```python
from build123d import *

# Parameters (mm, degrees)
BOSS_EXTRUDE1_DEPTH = 2
CHAMFER3_SIZE       = 0.2
SKETCH4_R           = 1
SKETCH4_R_2         = 2
CUT_EXTRUDE3_DEPTH  = 2
CHAMFER5_SIZE       = 0.1
CHAMFER6_SIZE       = 0.1


with BuildPart() as part:
    # Sketch1 → Boss-Extrude1 (new body)
    with BuildSketch(Plane.XY):
        with BuildLine():
            Line((-18, 3), (18, 3))
            ThreePointArc((18, 3), (21, 0), (18, -3))
            Line((18, -3), (-18, -3))
            ThreePointArc((-18, -3), (-21, 0), (-18, 3))
        make_face()
    extrude(amount=BOSS_EXTRUDE1_DEPTH)

    # Chamfer3
    chamfer3_edges = [part.edges().sort_by_distance(p)[0] for p in [
        (21, 0, 2),
        (0, 3, 2),
        (-21, 0, 2),
        (0, 3, 0),
        (21, 0, 0),
        (0, -3, 0),
        (-21, 0, 0),
        (0, -3, 2),
    ]]
    chamfer(chamfer3_edges, length=CHAMFER3_SIZE)

    # Sketch4 → Cut-Extrude3 (cut)
    with BuildSketch(Plane.XY.offset(2)):
        with Locations((-18, 0)):
            Circle(SKETCH4_R)
        with Locations((-12, 0)):
            Circle(SKETCH4_R_2)
        with Locations((-4, 0)):
            Circle(SKETCH4_R_2)
        with Locations((4, 0)):
            Circle(SKETCH4_R_2)
        with Locations((12, 0)):
            Circle(SKETCH4_R_2)
        with Locations((18, 0)):
            Circle(SKETCH4_R)
    extrude(amount=-CUT_EXTRUDE3_DEPTH, mode=Mode.SUBTRACT)

    # Chamfer5
    chamfer5_edges = [part.edges().sort_by_distance(p)[0] for p in [
        (-19, 0, 2),
        (-6, 0, 2),
        (-14, 0, 2),
        (2, 0, 2),
        (10, 0, 2),
        (17, 0, 2),
    ]]
    chamfer(chamfer5_edges, length=CHAMFER5_SIZE)

    # Chamfer6
    chamfer6_edges = [part.edges().sort_by_distance(p)[0] for p in [
        (-19, 0, 0),
        (-6, 0, 0),
        (-14, 0, 0),
        (2, 0, 0),
        (10, 0, 0),
        (17, 0, 0),
    ]]
    chamfer(chamfer6_edges, length=CHAMFER6_SIZE)


solid = part.part
```
Input: part model. Units: mm. Frame: model coordinates. Give positions to 0.01 mm unless a question says otherwise; leave off trailing zeros. Order: outer loops, then holes, each group sorted by start corner. A loop starts at its lowest first (then second) coordinate and runs counter-clockwise, first axis right, second up. Notation, with made-up numbers: M -28,4.5 L 11,4.5 A23 ccw 11,30.5 Z; hole C 65.25,30 d6. An arc over 180 degrees is marked long. Return JSON: item names as keys, results as strings.
Item 1: Cut plane A-A (x = -12). Return loops of the section in (y, z).
Solutions:
{"outline": "M -3,0.2 L -2.8,0 L -2.1,0 L -2,0.1 L -2,1.9 L -2.1,2 L -2.8,2 L -3,1.8 Z; M 2,0.1 L 2.1,0 L 2.8,0 L 3,0.2 L 3,1.8 L 2.8,2 L 2.1,2 L 2,1.9 Z"}
Item 2: Pull-direction query (Y, two-part tool) for faces 1 (the cylindrical face through (21, 0, 1)), 2 (the flat face through (0, 0, 0)), 3 (the cylindrical face through (-13.6, -1.2, 1)); classes: +Y half, -Y half, draft (parallel to the pull), parting line (faces both ways), or undercut.
Solutions:
{"face 1": "parting line", "face 2": "draft", "face 3": "undercut"}
Item 3: Cut plane C-C (y = 0). State how many separate pieces and enclosed holes the cut face has, then the cut area to 3 significant figures.
Solutions:
{"separate pieces": "7", "enclosed holes": "0", "area": "43.8 mm^2"}
Item 4: Cut plane B-B (z = 0.85). Return loops of the section in (x, y).
Solutions:
{"outline": "M -18,-3 L 18,-3 A3 ccw 18,3 L -18,3 A3 ccw Z; hole C -18,0 d2; hole C -12,0 d4; hole C -4,0 d4; hole C 4,0 d4; hole C 12,0 d4; hole C 18,0 d2"}
Item 5: Ray query, probe 1 along Y at (x, z) = (4, 0.7); probe 2 along Y at (x, z) = (-18, 1.2); probe 3 along X at (y, z) = (1.8, 1.05). Return the intervals inside material, ascending.
Solutions:
{"probe 1": "-3 to -2, 2 to 3", "probe 2": "-3 to -1, 1 to 3", "probe 3": "-20.4 to -12.87, -11.13 to -4.87, -3.13 to 3.13, 4.87 to 11.13, 12.87 to 20.4"}
